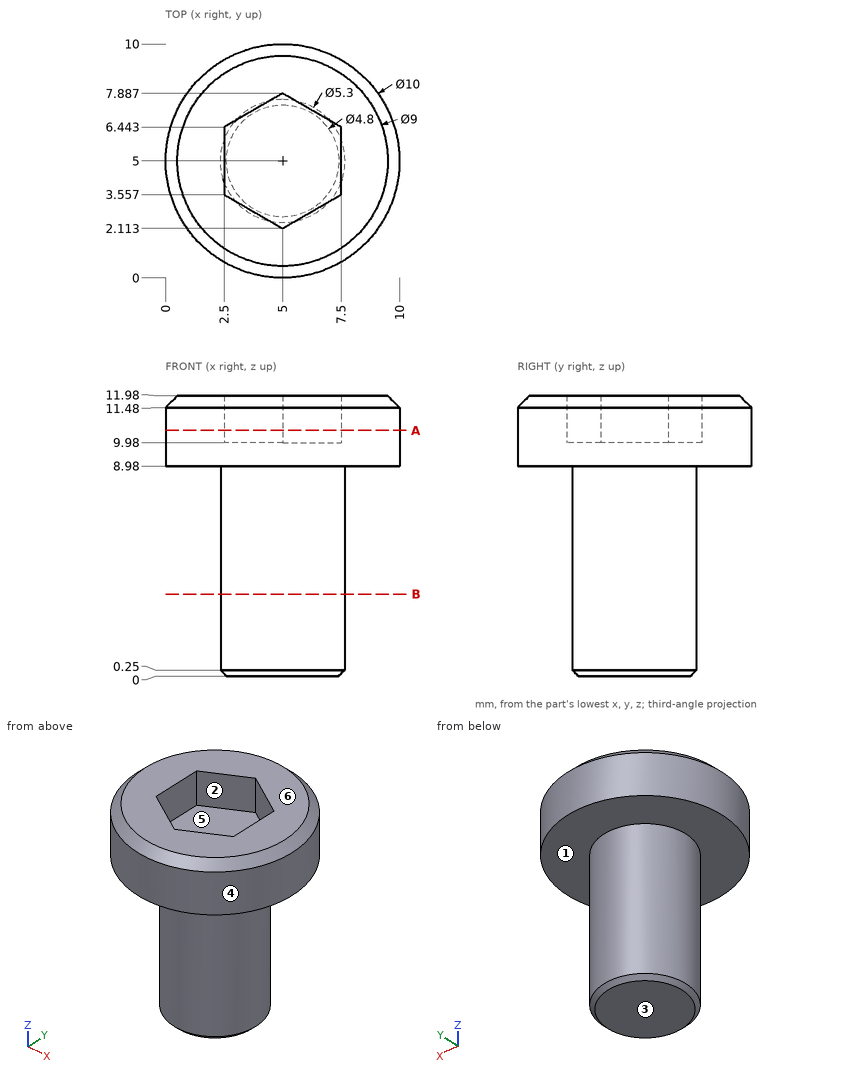
For this review, use the dimensioned drawing (mm, ordinates from the lowest corner) and the shaded views. A direction names the side the tool comes from. Give positions to 0.01 mm unless a question says otherwise; leave off trailing zeros. Loops run counter-clockwise (first coordinate to the right, second up) from the corner with the lowest first, then second, coordinate; pieces in that order, holes last.
Item 1: Tool access review of the marked faces 1, 2 and 3: name each direction out of +Z, -Z, +X, -X, +Y, -Y from which nothing blocks a thin tool from reaching the whole face with its end or side.
Item 2: Draft analysis for pull direction X (two halves, no side actions). For the marked faces 4, 5 and 6, state which applies: +X half, -X half, draft (parallel to the pull), parting line (faces both ways), or undercut.
Item 3: For line 1 along Z through (x, y) = (6.25, 4.5); line 2 along X through (y, z) = (5, 1.5); line 3 along Z through (x, y) = (6, 9), list the stretches that pass through material, from the lowest coordinate up.
Item 4: Take a section at B-B, the plane z = 3.5. State the section outline as (x, y) points.
Item 5: Take a section at A-A, the plane z = 10.5. State the section outline as (x, y) points, and give its area (3 significant figures).
Item 6: Insertion check: pin 1 (1.5 mm diameter, centred on x = 4.5, z = 7.5, fed in from -Y); pin 2 (1.5 mm diameter, centred on x = 6.5, z = 2.5, fed in from -Y); pin 3 (3 mm diameter, centred on y = 5, z = 4, fed in from +X). Each pin has a flat end and moves straight along its axis. Give the tip position at first contact, or say it passes through.
Calculated:
1. face 1: -Z
1. face 2: +Z
1. face 3: -Z, +X, -X, +Y, -Y
2. face 4: parting line
2. face 5: undercut
2. face 6: draft
3. line 1: z = 0 to 9.98
3. line 2: x = 2.35 to 7.65
3. line 3: z = 8.98 to 11.98
4. outline: circle Ø5.3 at (5, 5)
5. outline: circle Ø10 at (5, 5); hole (2.5, 3.56) - (5, 2.11) - (7.5, 3.56) - (7.5, 6.44) - (5, 7.89) - (2.5, 6.44) - close
5. area: 56.9 mm2
6. pin 1: stops at y = 2.35
6. pin 2: stops at y = 2.46
6. pin 3: stops at x = 7.65
